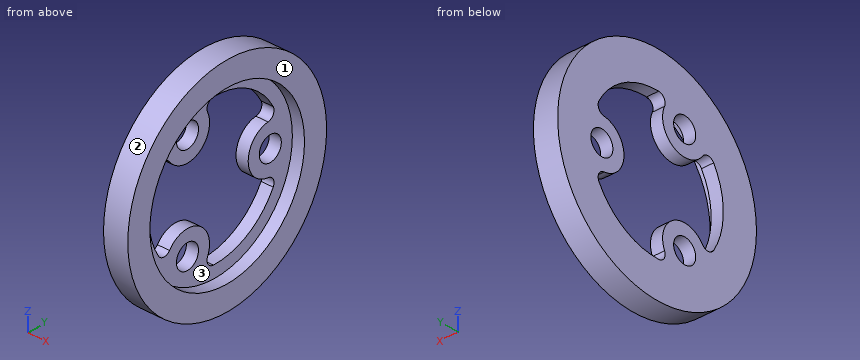
```python
from build123d import *

# Parameters (mm, degrees)
CROQUIS1_W            = 10
CROQUIS1_H            = 45
CROQUIS2_R            = 35
CORTAR_EXTRUIR1_DEPTH = 5
CROQUIS4_R            = 5
CORTAR_EXTRUIR3_DEPTH = 5


with BuildPart() as part:
    # Croquis1 → Revolución1 (revolve)
    with BuildSketch(Plane.XY, mode=Mode.PRIVATE) as revoluci_n1_sk:
        with Locations((5, 22.5)):
            Rectangle(CROQUIS1_W, CROQUIS1_H)
    revolve(revoluci_n1_sk.sketch.rotate(Axis((0, 0, 0), (1, 0, 0)), 180), axis=Axis((0, 0, 0), (1, 0, 0)))

    # Croquis2 → Cortar-Extruir1 (cut)
    with BuildSketch(Plane(origin=(10, 0, 0), x_dir=(0, 0, -1), z_dir=(1, 0, 0))):
        with Locations(Location((0, 0, 0), (0, 0, 90))):
            Circle(CROQUIS2_R)
    extrude(amount=-CORTAR_EXTRUIR1_DEPTH, mode=Mode.SUBTRACT)

    # Croquis4 → Cortar-Extruir3 (cut)
    with BuildSketch(Plane(origin=(5, 0, 0), x_dir=(0, 0, -1), z_dir=(1, 0, 0))):
        with BuildLine():
            ThreePointArc((29.991356012, -0.720114266), (25.980762114, 15), (14.372040758, 26.333333333))
            ThreePointArc((14.372040758, 26.333333333), (11.534836682, 26.353299832), (9.949874371, 24))
            ThreePointArc((9.949874371, 24), (0, 15), (-9.949874371, 24))
            ThreePointArc((-9.949874371, 24), (-11.534836682, 26.353299832), (-14.372040758, 26.333333333))
            ThreePointArc((-14.372040758, 26.333333333), (-25.980762114, 15), (-29.991356012, -0.720114266))
            ThreePointArc((-29.991356012, -0.720114266), (-28.590045469, -3.187188321), (-25.759546876, -3.38315603))
            ThreePointArc((-25.759546876, -3.38315603), (-12.990381057, -7.5), (-15.809672505, -20.61684397))
            ThreePointArc((-15.809672505, -20.61684397), (-17.055208787, -23.166111512), (-15.619315254, -25.613219068))
            ThreePointArc((-15.619315254, -25.613219068), (0, -30), (15.619315254, -25.613219067))
            ThreePointArc((15.619315254, -25.613219067), (17.055208787, -23.166111512), (15.809672505, -20.61684397))
            ThreePointArc((15.809672505, -20.61684397), (12.990381057, -7.5), (25.759546876, -3.38315603))
            ThreePointArc((25.759546876, -3.38315603), (28.59004547, -3.187188321), (29.991356012, -0.720114266))
        make_face()
        with Locations(Location((0, 25, 0), (0, 0, 90))):
            Circle(CROQUIS4_R)
        with Locations(Location((21.650635095, -12.5, 0), (0, 0, 90))):
            Circle(CROQUIS4_R)
        with Locations(Location((-21.650635095, -12.5, 0), (0, 0, 90))):
            Circle(CROQUIS4_R)
    extrude(amount=-CORTAR_EXTRUIR3_DEPTH, mode=Mode.SUBTRACT)


solid = part.part
```
For this review, take the finished solid that the model builds, in its own axes (mm). Face numbers are marked on the shaded views. Round coordinates to 2 decimals unless told otherwise and drop trailing zeros. Write each loop counter-clockwise with the first axis right and the second up, starting at its lowest first coordinate (ties: lowest second). Pieces come first, ordered by that corner, then holes. Notation, with made-up numbers: (43, 73) -> (61, 73) arc R28 ccw to (61, 109) -> close; hole circle Ø2 at (75.5, 89). An arc over 180 degrees is marked (long way). Use one line per item in the form item = value.
1) Take a section at C-C, the plane z = -28. Write out the cut boundary in (x, y), and give its area (3 significant figures).
Found:
outline = (0, -35.23) -> (10, -35.23) -> (10, -21) -> (5, -21) -> (5, -3.47) -> (0, -3.47) -> close; (0, 10.77) -> (5, 10.77) -> (5, 21) -> (10, 21) -> (10, 35.23) -> (0, 35.23) -> close
area = 423 mm2
2) Mouldability with a two-part tool opening along Y and no side actions: class the marked faces 1, 2 and 3 as +Y half, -Y half, draft (parallel to the pull), parting line (faces both ways), or undercut.
Found:
face_1 = draft
face_2 = parting line
face_3 = undercut
3) Take a section at A-A, the plane z = 0. Write out the cut boundary in (x, y).
Found:
outline = (0, -45) -> (10, -45) -> (10, -35) -> (5, -35) -> (5, -30) -> (0, -30) -> close; (0, 15) -> (5, 15) -> (5, 20) -> (0, 20) -> close; (0, 30) -> (5, 30) -> (5, 35) -> (10, 35) -> (10, 45) -> (0, 45) -> close
4) Take a section at D-D, the plane y = -28.5. Write out the cut boundary in (x, z), and give its area (3 significant figures).
Found:
outline = (0, -34.82) -> (10, -34.82) -> (10, -20.32) -> (5, -20.32) -> (5, -9.37) -> (0, -9.37) -> close; (0, 9.37) -> (5, 9.37) -> (5, 20.32) -> (10, 20.32) -> (10, 34.82) -> (0, 34.82) -> close
area = 400 mm2
5) Take a section at B-B, the plane y = -12.5. Write out the cut boundary in (x, z).
Found:
outline = (0, -43.23) -> (10, -43.23) -> (10, -32.69) -> (5, -32.69) -> (5, -26.65) -> (0, -26.65) -> close; (0, -16.65) -> (5, -16.65) -> (5, -11.65) -> (0, -11.65) -> close; (0, 11.65) -> (5, 11.65) -> (5, 16.65) -> (0, 16.65) -> close; (0, 26.65) -> (5, 26.65) -> (5, 32.69) -> (10, 32.69) -> (10, 43.23) -> (0, 43.23) -> close
6) Clearance check with flat-ended pins moving along their axes: pin 1 (10 mm diameter, centred on y = -20, z = -23, fed in from +X); pin 2 (5 mm diameter, centred on x = 4.5, y = 3.5, fed in from -Z); pin 3 (1 mm diameter, centred on x = 7.5, y = -33, fed in from -Z); pin 4 (4 mm diameter, centred on x = 2, y = 33, fed in from -Z). State where each tip first meets the part, or that it passes through.
Found:
pin_1 = 10
pin_2 = -44.99
pin_3 = -31.12
pin_4 = -32.62
7) To check wall thickness, follow L1, parallel to Z at x = 4, y = 21; L2, parallel to Z at x = 1.8, y = -12.5; L3, parallel to Z at x = 3.75, y = 29.5. State the ranges of each line that lie inside material, in increasing order. Write a range as from..to.
Found:
L1 = -39.8..-21.42, -9.17..-3, 3..9.17, 21.42..39.8
L2 = -43.23..-26.65, -16.65..-11.65, 11.65..16.65, 26.65..43.23
L3 = -33.98..-2.18, 2.18..33.98
